The listing builds one solid part. Answer for the finished solid, in the listing's coordinates (mm). A direction names the side the tool comes from. Round coordinates to 2 decimals unless told otherwise and drop trailing zeros.
(1) For faces 4 (the face through (-441, 13, -359.525)), 5 (the face through (600, 13, 6)), determine the directions among +Z, -Z, +X, -X, +Y, -Y from which every point of the face is accessible in a straight line to the end or side of a thin tool.
(2) The mould has two halves that part along Z. Classify faces 1 (the face through (-439, 13, 359.525)), 2 (the face through (-8, 13, 450)), 3 (the face through (-8, 0, -6)): +Z half, -Z half, draft (parallel to the pull), parting line (faces both ways), or undercut.
(3) Find the intervals of material crossed by probe 1 along Z at (x, y) = (-462.5, 3.25) (3 decimals), in increasing order.
from build123d import *

# Parameters (mm, degrees)
CROQUIS1_W              = 1200
CROQUIS1_H              = 900
SALIENTE_EXTRUIR1_DEPTH = 25.4
CORTAR_EXTRUIR1_DEPTH   = 25.4


with BuildPart() as part:
    # Croquis1 → Saliente-Extruir1 (new body)
    with BuildSketch(Plane(origin=(0, 0, 0), x_dir=(1, 0, 0), z_dir=(0, 1, 0))):
        Rectangle(CROQUIS1_W, CROQUIS1_H)
    extrude(amount=SALIENTE_EXTRUIR1_DEPTH)

    # Croquis2 → Cortar-Extruir1 (cut)
    with BuildSketch(Plane(origin=(0, 25.4, 0), x_dir=(1, 0, 0), z_dir=(0, 1, 0))):
        with BuildLine():
            Line((390, 359.525), (490, 359.525))
            ThreePointArc((490, 359.525), (499.525, 350), (490, 340.475))
            Line((490, 340.475), (390, 340.475))
            ThreePointArc((390, 340.475), (380.475, 350), (390, 359.525))
        make_face()
        with BuildLine():
            Line((-390, 340.475), (-490, 340.475))
            ThreePointArc((-490, 340.475), (-499.525, 350), (-490, 359.525))
            Line((-490, 359.525), (-390, 359.525))
            ThreePointArc((-390, 359.525), (-380.475, 350), (-390, 340.475))
        make_face()
        with BuildLine():
            Line((-390, -359.525), (-490, -359.525))
            ThreePointArc((-490, -359.525), (-499.525, -350), (-490, -340.475))
            Line((-490, -340.475), (-390, -340.475))
            ThreePointArc((-390, -340.475), (-380.475, -350), (-390, -359.525))
        make_face()
        with BuildLine():
            Line((390, -340.475), (490, -340.475))
            ThreePointArc((490, -340.475), (499.525, -350), (490, -359.525))
            Line((490, -359.525), (390, -359.525))
            ThreePointArc((390, -359.525), (380.475, -350), (390, -340.475))
        make_face()
    extrude(amount=-CORTAR_EXTRUIR1_DEPTH, mode=Mode.SUBTRACT)


solid = part.part
Solutions:
1. face 4: +Y, -Y
1. face 5: +Z, -Z, +X, +Y, -Y
2. face 1: undercut
2. face 2: +Z half
2. face 3: draft
3. probe 1: z = -450 to -359.525, -340.475 to 340.475, 359.525 to 450
